Answer from the drawing. Dimensions are ordinates in mm from the lowest x, y and z of the part. Coordinates: 2 decimals unless noted, no trailing zeros. Write each loop counter-clockwise with the first axis right and the second up, starting at its lowest first coordinate (ties: lowest second). Pieces come first, ordered by that corner, then holes. Notation, with made-up numbers: (52, 49) -> (67, 49) arc R24 cw to (67, 70) -> close; hole circle Ø8 at (87.5, -12). An arc over 180 degrees is marked (long way). Use CSV: the item, a comma, the result in double quotes.
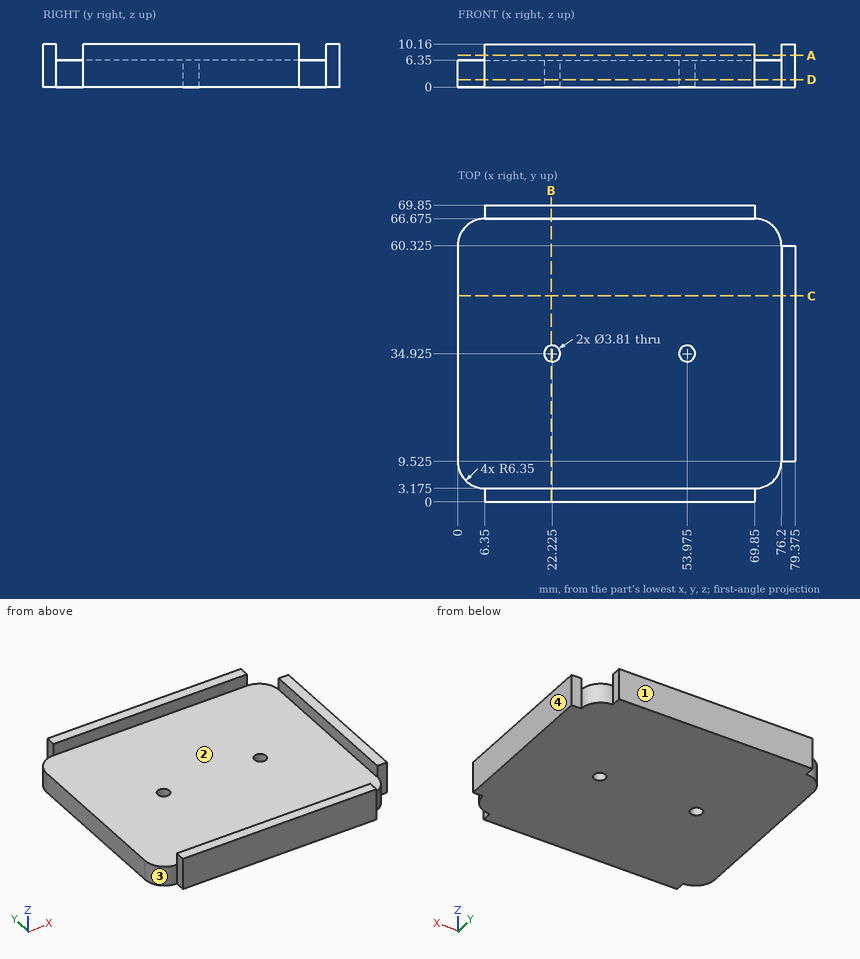
1. For a pull along Y with two mould halves and no side action, classify the marked faces 1, 2, 3 and 4 as pulls with the +Y half, pulls with the -Y half, needs draft (parallel to the pull), parting line crosses it, or undercut.
Solutions:
face 1,"pulls with the +Y half"
face 2,"undercut"
face 3,"pulls with the -Y half"
face 4,"needs draft"
2. A cutting plane is placed at B-B (x = 22). Give the vertices of the cut face in (y, z) (3 decimals).
Solutions:
outline,"(0, 0) -> (33.033, 0) -> (33.033, 6.35) -> (3.175, 6.35) -> (3.175, 10.16) -> (0, 10.16) -> close; (36.817, 0) -> (69.85, 0) -> (69.85, 10.16) -> (66.675, 10.16) -> (66.675, 6.35) -> (36.817, 6.35) -> close"
3. Find the intervals of material crossed by line 1 along Y through (x, z) = (42.5, 7.5) (3 decimals); line 2 along X through (y, z) = (57, 8) (3 decimals); line 3 along Z through (x, y) = (54, 54), in increasing order.
Solutions:
line 1,"y = 0 to 3.175, 66.675 to 69.85"
line 2,"x = 76.2 to 79.375"
line 3,"z = 0 to 6.35"
4. Each of these flat-tipped pins is pushed along its axis until it touches: pin 1 Ø4 at (x, y) = (62, 39) entering from -Z; pin 2 Ø3.5 at (y, z) = (69, 7) entering from +X; pin 3 Ø3 at (x, y) = (53.975, 34.925) entering from +Z; pin 4 Ø1.6 at (x, z) = (77.5, 4.5) entering from -Y (3 decimals). Where does it stop, or does it pass through?
Solutions:
pin 1,"stops at z = 0"
pin 2,"stops at x = 69.85"
pin 3,"passes through"
pin 4,"stops at y = 9.525"
5. A cutting plane is placed at C-C (y = 48.5). Give the vertices of the cut face in (x, z) (3 decimals).
Solutions:
outline,"(0, 0) -> (79.375, 0) -> (79.375, 10.16) -> (76.2, 10.16) -> (76.2, 6.35) -> (0, 6.35) -> close"
6. A cutting plane is placed at D-D (z = 1.75). Give the vertices of the cut face in (x, y) (3 decimals), and give its area (3 significant figures).
Solutions:
outline,"(0, 9.525) arc R6.35 ccw to (6.35, 3.175) -> (6.35, 0) -> (69.85, 0) -> (69.85, 3.175) arc R6.35 ccw to (76.2, 9.525) -> (79.375, 9.525) -> (79.375, 60.325) -> (76.2, 60.325) arc R6.35 ccw to (69.85, 66.675) -> (69.85, 69.85) -> (6.35, 69.85) -> (6.35, 66.675) arc R6.35 ccw to (0, 60.325) -> close; hole circle Ø3.81 at (22.225, 34.925); hole circle Ø3.81 at (53.975, 34.925)"
area,"5,350 mm^2"
7. A cutting plane is placed at A-A (z = 7.5). Give the vertices of the cut face in (x, y) (3 decimals), and give its area (3 significant figures).
Solutions:
outline,"(6.35, 0) -> (69.85, 0) -> (69.85, 3.175) -> (6.35, 3.175) -> close; (6.35, 66.675) -> (69.85, 66.675) -> (69.85, 69.85) -> (6.35, 69.85) -> close; (76.2, 9.525) -> (79.375, 9.525) -> (79.375, 60.325) -> (76.2, 60.325) -> close"
area,"565 mm^2"
